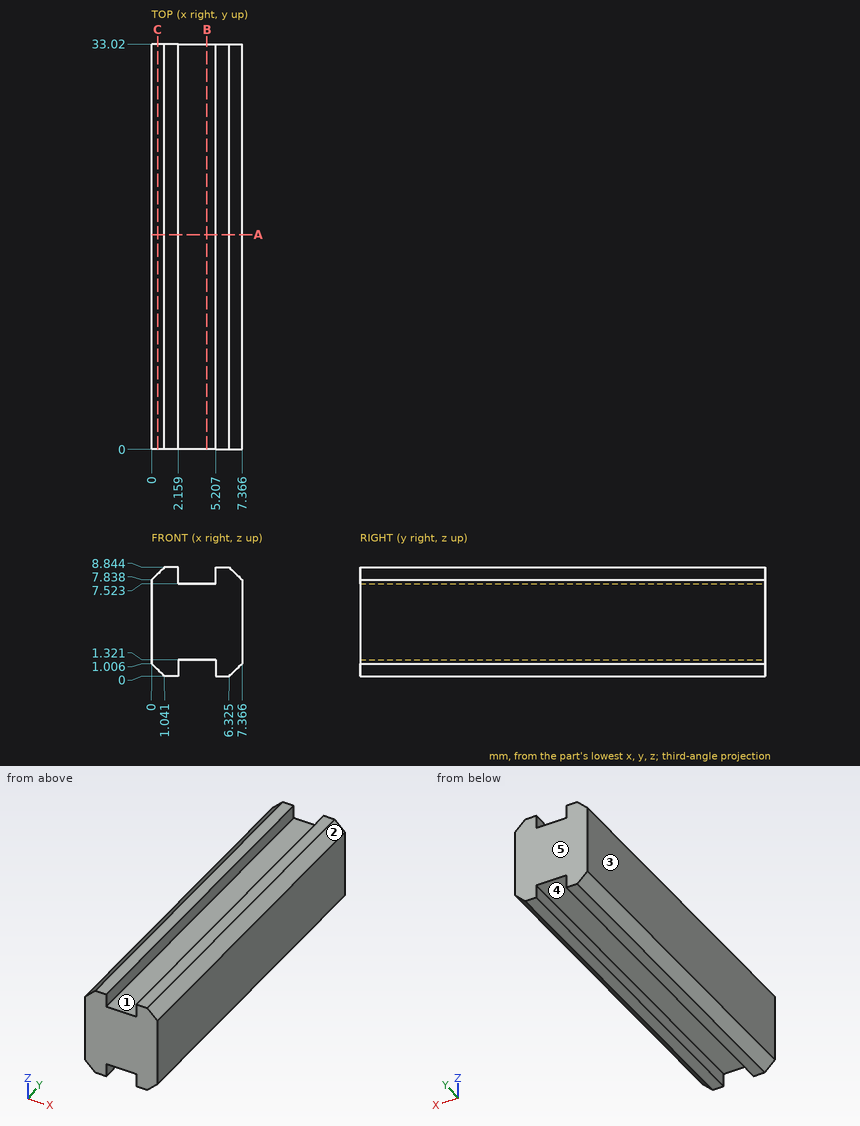
Study the drawing (mm; zero at the part's minimum x, y, z) and answer. A direction names the side the tool comes from. Give positions to 0.01 mm unless a question says otherwise; leave off trailing zeros. Loops run counter-clockwise (first coordinate to the right, second up) from the corner with the lowest first, then second, coordinate; pieces in that order, holes last. Notation, with made-up numbers: (70.5, 7) - (107.5, 7) arc R28 cw to (107.5, 30) - close; hole circle Ø3 at (-35.75, -0.75). An arc over 180 degrees is marked (long way). Answer in a Markdown table with one row per item. Add a question column.
Q1. A tool of negligible diameter and unlimited length cuts with its end or side. For the marked faces 4 and 5, from which of +Z, -Z, +X, -X, +Y, -Y can it reach the whole face along a straight path? Write none if from no direction.
Q2. Determine the mould class of the marked faces 1, 2 and 3 for opening direction X: released by +X, released by -X, zero draft, split by the parting line, or undercut.
Q3. The part is cut by section A-A (y = 17.5). Determine the outline of the cut face in (x, z) (1 decimal), and give its area (3 significant figures).
Q4. Each of these flat-tipped pins is pushed along its axis until it touches: P1, Ø2.5, axis at x = 3.5, y = 13, coming from the -Z side; P2, Ø1.1, axis at y = 19, z = 8.5, coming from the -X side (1 decimal); P3, Ø2.5, axis at x = 3.5, y = 20.5, coming from the +Z side. Where does it stop, or does it pass through?
Q5. The part is cut by section B-B (x = 4.5). Determine the outline of the cut face in (y, z), and give its area (3 significant figures).
Q6. The part is cut by section C-C (x = 0.5). Determine the outline of the cut face in (y, z).
Q7. Consider line 1 along X through (y, z) = (25, 7.75); line 2 along Z through (x, y) = (3.25, 28); line 3 along X through (y, z) = (22.5, 8.5) (1 decimal). Determine where each line is inside the solid, lowest interval first.
Solution:
| question | item | result |
|---|---|---|
| 1 | face 4 | -Z, +Y, -Y |
| 1 | face 5 | +Z, -Z, +X, -X, +Y |
| 2 | face 1 | undercut |
| 2 | face 2 | released by +X |
| 2 | face 3 | released by -X |
| 3 | outline | (0, 1) - (1, 0) - (2.2, 0) - (2.2, 1.3) - (5.2, 1.3) - (5.2, 0) - (6.3, 0) - (7.4, 1) - (7.4, 7.8) - (6.3, 8.8) - (5.2, 8.8) - (5.2, 7.5) - (2.2, 7.5) - (2.2, 8.8) - (1, 8.8) - (0, 7.8) - close |
| 3 | area | 55.0 mm² |
| 4 | P1 | stops at z = 1.32 |
| 4 | P2 | stops at x = 0.1 |
| 4 | P3 | stops at z = 7.52 |
| 5 | outline | (0, 1.32) - (33.02, 1.32) - (33.02, 7.52) - (0, 7.52) - close |
| 5 | area | 205 mm² |
| 6 | outline | (0, 0.52) - (33.02, 0.52) - (33.02, 8.32) - (0, 8.32) - close |
| 7 | line 1 | x = 0 to 2.16, 5.21 to 7.37 |
| 7 | line 2 | z = 1.32 to 7.52 |
| 7 | line 3 | x = 0.7 to 2.2, 5.2 to 6.7 |
